from build123d import *

# Parameters (mm, degrees)
SKETCH_1_W          = 67.85270183
SKETCH_1_H          = 67.85270183
EXTRUDE_1_DEPTH     = 17
SKETCH_2_R          = 11
CUT_EXTRUDE_1_DEPTH = 17
SKETCH_3_R          = 2
CUT_EXTRUDE_2_DEPTH = 17


with BuildPart() as part:
    # 草图1 → 凸台-拉伸1 (new body)
    with BuildSketch(Plane.XY):
        with Locations((-0.966617145, 2.637078742)):
            Rectangle(SKETCH_1_W, SKETCH_1_H)
    extrude(amount=-EXTRUDE_1_DEPTH)

    # 草图2 → 切除-拉伸1 (cut)
    with BuildSketch(Plane.XY):
        Circle(SKETCH_2_R)
    extrude(amount=-CUT_EXTRUDE_1_DEPTH, mode=Mode.SUBTRACT)

    # 草图3 → 切除-拉伸2 (cut)
    with BuildSketch(Plane.XY):
        with Locations((-15.5, 15.5)):
            Circle(SKETCH_3_R)
        with Locations((15.5, 15.5)):
            Circle(SKETCH_3_R)
        with Locations((-15.5, -15.5)):
            Circle(SKETCH_3_R)
        with Locations((15.5, -15.5)):
            Circle(SKETCH_3_R)
    extrude(amount=-CUT_EXTRUDE_2_DEPTH, mode=Mode.SUBTRACT)


solid = part.part
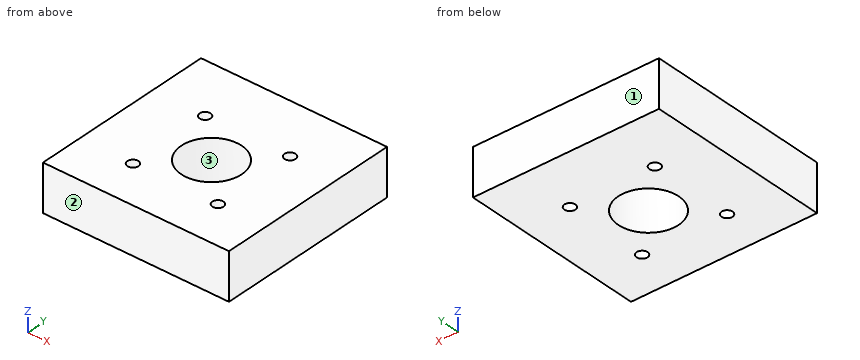
Build history of the part. All positions in model axes, mm. Face numbers are marked on the shaded views. Round coordinates to 2 decimals unless told otherwise and drop trailing zeros. Write each loop counter-clockwise with the first axis right and the second up, starting at its lowest first coordinate (ties: lowest second). Pieces come first, ordered by that corner, then holes. Notation, with made-up numbers: (25.5, 54) -> (29.5, 54) arc R18 cw to (29.5, 77) -> close; hole circle Ø10 at (17.25, 49). An arc over 180 degrees is marked (long way). Write item = value, one per line.
(1) Probe L1, parallel to Y at x = 15.5, z = -6.75; L2, parallel to X at y = -16, z = -13; L3, parallel to X at y = -16.5, z = -9. List the from-to ranges inside material, lowest first.
Answer:
L1 = -31.29 to -17.5, -13.5 to 13.5, 17.5 to 36.56
L2 = -34.89 to -17.44, -13.56 to 13.56, 17.44 to 32.96
L3 = -34.89 to -17.23, -13.77 to 13.77, 17.23 to 32.96
(2) Band-saw the part on D-D (x = -15.5). Give the cut face in (y, z), then the cut area to 3 significant figures.
Answer:
outline = (-31.29, -17) -> (-17.5, -17) -> (-17.5, 0) -> (-31.29, 0) -> close; (-13.5, -17) -> (13.5, -17) -> (13.5, 0) -> (-13.5, 0) -> close; (17.5, -17) -> (36.56, -17) -> (36.56, 0) -> (17.5, 0) -> close
area = 1,020 mm2
(3) Two-plate mould, pull along Y, no slides. Class the marked faces 1, 2 and 3: pulls with the +Y half, pulls with the -Y half, needs draft (parallel to the pull), parting line crosses it, or undercut.
Answer:
face_1 = pulls with the +Y half
face_2 = pulls with the -Y half
face_3 = undercut
(4) Band-saw the part on B-B (y = 0). Give the cut face in (x, z), then the cut area to 3 significant figures.
Answer:
outline = (-34.89, -17) -> (-11, -17) -> (-11, 0) -> (-34.89, 0) -> close; (11, -17) -> (32.96, -17) -> (32.96, 0) -> (11, 0) -> close
area = 779 mm2
(5) Band-saw the part on A-A (y = 15.5). Give the cut face in (x, z), then the cut area to 3 significant figures.
Answer:
outline = (-34.89, -17) -> (-17.5, -17) -> (-17.5, 0) -> (-34.89, 0) -> close; (-13.5, -17) -> (13.5, -17) -> (13.5, 0) -> (-13.5, 0) -> close; (17.5, -17) -> (32.96, -17) -> (32.96, 0) -> (17.5, 0) -> close
area = 1,020 mm2
(6) Band-saw the part on C-C (z = -12.5). Give the cut face in (x, y).
Answer:
outline = (-34.89, -31.29) -> (32.96, -31.29) -> (32.96, 36.56) -> (-34.89, 36.56) -> close; hole circle Ø4 at (-15.5, -15.5); hole circle Ø4 at (-15.5, 15.5); hole circle Ø22 at (0, 0); hole circle Ø4 at (15.5, -15.5); hole circle Ø4 at (15.5, 15.5)
